Could you check a few things on this model? Use its own coordinates, in mm. A direction names the side the tool comes from. Coordinates: 2 decimals unless noted, no trailing zeros. Loops run counter-clockwise (first coordinate to the right, second up) from the corner with the lowest first, then second, coordinate; pieces in that order, holes last.
1) If I drill on line 1 along Y through (x, z) = (-6.35, -8.3) (3 decimals); line 2 along Z through (x, y) = (-7.5, -4.75); line 3 along X through (y, z) = (1.5, 4.75), over which ranges is the centre line in solid material (lowest first)?
2) Imagine slicing it at C-C on z = 4.5. Please give me the cut outline in (x, y), plus the area to 3 significant figures.
3) Thinking about a two-plate mould opening in Y: for faces 6 (the face through (-3, -2, 8.89)), 7 (the face through (-3.32, 0.95, -7.86)), 8 (the face through (2, -8.89, 0)), which applies, released by +Y, released by -Y, zero draft, split by the parting line, or undercut?
4) Imagine slicing it at A-A on x = -6.35. Please give me the cut outline in (y, z) (3 decimals), plus the area to 3 significant figures.
5) Imagine slicing it at D-D on y = 7.75. Please give me the cut outline in (x, z).
6) Will these pins go through, and if not, where does the flat tip stop? P1, Ø4, axis at x = -6.35, y = 0, coming from the +Z side; P2, Ø8, axis at x = 47, y = -7, coming from the +Z side; P3, Ø8, axis at x = 8.5, z = 2.5, coming from the +Y side; P4, Ø7, axis at y = 0.5, z = 2, coming from the -X side.
7) For faces 1 (the face through (-9.1, -1.9, -6.858)), 2 (the face through (2.54, -7, -7)), 3 (the face through (2.54, 7, 7)), 4 (the face through (2.54, 7, -7)), 5 (the face through (2.54, -7, 7)), which set-ups out of +Z, -Z, +X, -X, +Y, -Y let a thin tool reach every point of the face, with its end or its side?
8) Imagine slicing it at B-B on y = -6.75. Please give me the cut outline in (x, z), plus the area to 3 significant figures.
```python
from build123d import *

# Parameters (mm, degrees)
SKETCH2_W           = 17.78
SKETCH2_H           = 17.78
BOSS_EXTRUDE1_DEPTH = 2.54
SKETCH3_R           = 8.89
BOSS_EXTRUDE2_DEPTH = 63.5
SKETCH4_W           = 17.78
SKETCH4_H           = 2.032
BOSS_EXTRUDE3_DEPTH = 12.7
SKETCH5_R           = 3.175
CUT_EXTRUDE1_DEPTH  = 69.966963831


with BuildPart() as part:
    # Sketch2 → Boss-Extrude1 (new body)
    with BuildSketch(Plane.YZ):
        Rectangle(SKETCH2_W, SKETCH2_H)
    extrude(amount=BOSS_EXTRUDE1_DEPTH)

    # Sketch3 → Boss-Extrude2 (add)
    with BuildSketch(Plane(origin=(2.54, 0, 0), x_dir=(0, 0, -1), z_dir=(1, 0, 0))):
        Circle(SKETCH3_R)
    extrude(amount=BOSS_EXTRUDE2_DEPTH)

    # Sketch4 → Boss-Extrude3 (add)
    with BuildSketch(Plane(origin=(0, 0, 0), x_dir=(0, -1, 0), z_dir=(-1, 0, 0))):
        with Locations((0, 7.874)):
            Rectangle(SKETCH4_W, SKETCH4_H)
        with Locations((0, -7.874)):
            Rectangle(SKETCH4_W, SKETCH4_H)
    extrude(amount=BOSS_EXTRUDE3_DEPTH)

    # Sketch5 → Cut-Extrude1 (cut, through all)
    with BuildSketch(Plane.XY.offset(8.89)):
        with Locations((-6.35, 0)):
            Circle(SKETCH5_R)
    extrude(amount=-CUT_EXTRUDE1_DEPTH, mode=Mode.SUBTRACT)


solid = part.part
```
Filled in:
1. line 1: y = -8.89 to -3.175, 3.175 to 8.89
1. line 2: z = -8.89 to -6.86, 6.86 to 8.89
1. line 3: x = 0 to 66.04
2. outline: (0, -8.89) - (2.54, -8.89) - (2.54, -7.67) - (66.04, -7.67) - (66.04, 7.67) - (2.54, 7.67) - (2.54, 8.89) - (0, 8.89) - close
2. area: 1,020 mm2
3. face 6: zero draft
3. face 7: undercut
3. face 8: released by -Y
4. outline: (-8.89, -8.89) - (-3.175, -8.89) - (-3.175, -6.858) - (-8.89, -6.858) - close; (-8.89, 6.858) - (-3.175, 6.858) - (-3.175, 8.89) - (-8.89, 8.89) - close; (3.175, -8.89) - (8.89, -8.89) - (8.89, -6.858) - (3.175, -6.858) - close; (3.175, 6.858) - (8.89, 6.858) - (8.89, 8.89) - (3.175, 8.89) - close
4. area: 46.5 mm2
5. outline: (-12.7, -8.89) - (2.54, -8.89) - (2.54, -4.36) - (66.04, -4.36) - (66.04, 4.36) - (2.54, 4.36) - (2.54, 8.89) - (-12.7, 8.89) - (-12.7, 6.86) - (0, 6.86) - (0, -6.86) - (-12.7, -6.86) - close
6. P1: passes through
6. P2: stops at z = 8.37
6. P3: stops at y = 8.89
6. P4: stops at x = 0
7. face 1: -X, +Y, -Y
7. face 2: -Z, +X, -Y
7. face 3: +Z, +X, +Y
7. face 4: -Z, +X, +Y
7. face 5: +Z, +X, -Y
8. outline: (-12.7, -8.89) - (2.54, -8.89) - (2.54, -5.79) - (66.04, -5.79) - (66.04, 5.79) - (2.54, 5.79) - (2.54, 8.89) - (-12.7, 8.89) - (-12.7, 6.86) - (0, 6.86) - (0, -6.86) - (-12.7, -6.86) - close
8. area: 832 mm2
